```python
from build123d import *

# Parameters (mm, degrees)
SKETCH1_R                 = 1.5
SKETCH1_R_2               = 2.5
BATTERY_MOUNT_PLATE_DEPTH = 2.5
BATTERY_STRAP_SLOTS_DEPTH = 10
CUT_EXTRUDE1_DEPTH        = 10


with BuildPart() as part:
    # Sketch1 → battery mount plate (new body)
    with BuildSketch(Plane(origin=(0, 0, 0), x_dir=(1, 0, 0), z_dir=(0, 1, 0))):
        with BuildLine():
            Line((-145, 86), (145, 86))
            ThreePointArc((145, 86), (159.142135624, 80.142135624), (165, 66))
            Line((165, 66), (165, -66))
            ThreePointArc((165, -66), (159.142135624, -80.142135624), (145, -86))
            Line((145, -86), (-145, -86))
            ThreePointArc((-145, -86), (-159.142135624, -80.142135624), (-165, -66))
            Line((-165, -66), (-165, 66))
            ThreePointArc((-165, 66), (-159.142135624, 80.142135624), (-145, 86))
        make_face()
        with Locations(Location((143, 64, 0), (0, 0, 270))):
            Circle(SKETCH1_R, mode=Mode.SUBTRACT)
        with Locations(Location((-143, 64, 0), (0, 0, 90))):
            Circle(SKETCH1_R, mode=Mode.SUBTRACT)
        with Locations(Location((143, -64, 0), (0, 0, 90))):
            Circle(SKETCH1_R, mode=Mode.SUBTRACT)
        with Locations(Location((-143, -64, 0), (0, 0, 270))):
            Circle(SKETCH1_R, mode=Mode.SUBTRACT)
        with Locations(Location((-143, 20, 0), (0, 0, 270))):
            Circle(SKETCH1_R_2, mode=Mode.SUBTRACT)
        with Locations(Location((-143, -20, 0), (0, 0, 90))):
            Circle(SKETCH1_R_2, mode=Mode.SUBTRACT)
        with Locations(Location((143, 20, 0), (0, 0, 90))):
            Circle(SKETCH1_R_2, mode=Mode.SUBTRACT)
        with Locations(Location((143, -20, 0), (0, 0, 270))):
            Circle(SKETCH1_R_2, mode=Mode.SUBTRACT)
    extrude(amount=BATTERY_MOUNT_PLATE_DEPTH)

    # Sketch2 → battery strap slots (cut)
    with BuildSketch(Plane(origin=(0, 2.5, 0), x_dir=(1, 0, 0), z_dir=(0, 1, 0))):
        with BuildLine():
            Line((-25, 73), (-125, 73))
            ThreePointArc((-125, 73), (-127, 71), (-125, 69))
            Line((-125, 69), (-25, 69))
            ThreePointArc((-25, 69), (-23, 71), (-25, 73))
        make_face()
        with BuildLine():
            ThreePointArc((25, 73), (23, 71), (25, 69))
            Line((25, 69), (125, 69))
            ThreePointArc((125, 69), (127, 71), (125, 73))
            Line((125, 73), (25, 73))
        make_face()
        with BuildLine():
            ThreePointArc((25, 59), (23, 57), (25, 55))
            Line((25, 55), (125, 55))
            ThreePointArc((125, 55), (127, 57), (125, 59))
            Line((125, 59), (25, 59))
        make_face()
        with BuildLine():
            Line((-25, 59), (-125, 59))
            ThreePointArc((-125, 59), (-127, 57), (-125, 55))
            Line((-125, 55), (-25, 55))
            ThreePointArc((-25, 55), (-23, 57), (-25, 59))
        make_face()
        with BuildLine():
            Line((-25, -55), (-125, -55))
            ThreePointArc((-125, -55), (-127, -57), (-125, -59))
            Line((-125, -59), (-25, -59))
            ThreePointArc((-25, -59), (-23, -57), (-25, -55))
        make_face()
        with BuildLine():
            ThreePointArc((25, -55), (23, -57), (25, -59))
            Line((25, -59), (125, -59))
            ThreePointArc((125, -59), (127, -57), (125, -55))
            Line((125, -55), (25, -55))
        make_face()
        with BuildLine():
            ThreePointArc((25, -69), (23, -71), (25, -73))
            Line((25, -73), (125, -73))
            ThreePointArc((125, -73), (127, -71), (125, -69))
            Line((125, -69), (25, -69))
        make_face()
        with BuildLine():
            Line((-25, -69), (-125, -69))
            ThreePointArc((-125, -69), (-127, -71), (-125, -73))
            Line((-125, -73), (-25, -73))
            ThreePointArc((-25, -73), (-23, -71), (-25, -69))
        make_face()
    extrude(amount=-BATTERY_STRAP_SLOTS_DEPTH, mode=Mode.SUBTRACT)

    # Sketch3 → Cut-Extrude1 (cut)
    with BuildSketch(Plane(origin=(0, 2.5, 0), x_dir=(1, 0, 0), z_dir=(0, 1, 0))):
        with BuildLine():
            Line((-125, 40.910721278), (-125, 12))
            ThreePointArc((-125, 12), (-124.414213562, 10.585786438), (-123, 10))
            Line((-123, 10), (-85.829072643, 10))
            ThreePointArc((-85.829072643, 10), (-83.937326245, 11.35092715), (-84.601191416, 13.578704435))
            Line((-84.601191416, 13.578704435), (-121.772118773, 42.489425712))
            ThreePointArc((-121.772118773, 42.489425712), (-123.878702892, 42.707351798), (-125, 40.910721278))
        make_face()
        with BuildLine():
            Line((-84.601191416, -13.578704435), (-121.772118773, -42.489425712))
            ThreePointArc((-121.772118773, -42.489425712), (-123.878702892, -42.707351798), (-125, -40.910721278))
            Line((-125, -40.910721278), (-125, -12))
            ThreePointArc((-125, -12), (-124.414213562, -10.585786438), (-123, -10))
            Line((-123, -10), (-85.829072643, -10))
            ThreePointArc((-85.829072643, -10), (-83.937326245, -11.35092715), (-84.601191416, -13.578704435))
        make_face()
        with BuildLine():
            Line((-25, -40.910721278), (-25, -12))
            ThreePointArc((-25, -12), (-25.585786438, -10.585786438), (-27, -10))
            Line((-27, -10), (-64.170927357, -10))
            ThreePointArc((-64.170927357, -10), (-66.062673755, -11.35092715), (-65.398808584, -13.578704435))
            Line((-65.398808584, -13.578704435), (-28.227881227, -42.489425712))
            ThreePointArc((-28.227881227, -42.489425712), (-26.121297108, -42.707351798), (-25, -40.910721278))
        make_face()
        with BuildLine():
            Line((-65.398808584, 13.578704435), (-28.227881227, 42.489425712))
            ThreePointArc((-28.227881227, 42.489425712), (-26.121297108, 42.707351798), (-25, 40.910721278))
            Line((-25, 40.910721278), (-25, 12))
            ThreePointArc((-25, 12), (-25.585786438, 10.585786438), (-27, 10))
            Line((-27, 10), (-64.170927357, 10))
            ThreePointArc((-64.170927357, 10), (-66.062673755, 11.35092715), (-65.398808584, 13.578704435))
        make_face()
        with BuildLine():
            Line((-99.654825771, 42.489425712), (-50.345174229, 42.489425712))
            ThreePointArc((-50.345174229, 42.489425712), (-48.453427831, 41.138498563), (-49.117293002, 38.910721278))
            Line((-49.117293002, 38.910721278), (-73.772118773, 19.734745678))
            ThreePointArc((-73.772118773, 19.734745678), (-75, 19.313450112), (-76.227881227, 19.734745678))
            Line((-76.227881227, 19.734745678), (-100.882706998, 38.910721278))
            ThreePointArc((-100.882706998, 38.910721278), (-101.546572169, 41.138498563), (-99.654825771, 42.489425712))
        make_face()
        with BuildLine():
            Line((-49.117293002, -38.910721278), (-73.772118773, -19.734745678))
            ThreePointArc((-73.772118773, -19.734745678), (-75, -19.313450112), (-76.227881227, -19.734745678))
            Line((-76.227881227, -19.734745678), (-100.882706998, -38.910721278))
            ThreePointArc((-100.882706998, -38.910721278), (-101.546572169, -41.138498563), (-99.654825771, -42.489425712))
            Line((-99.654825771, -42.489425712), (-50.345174229, -42.489425712))
            ThreePointArc((-50.345174229, -42.489425712), (-48.453427831, -41.138498563), (-49.117293002, -38.910721278))
        make_face()
        with BuildLine():
            Line((76.227881227, -19.734745678), (100.882706998, -38.910721278))
            ThreePointArc((100.882706998, -38.910721278), (101.546572169, -41.138498563), (99.654825771, -42.489425712))
            Line((99.654825771, -42.489425712), (50.345174229, -42.489425712))
            ThreePointArc((50.345174229, -42.489425712), (48.453427831, -41.138498563), (49.117293002, -38.910721278))
            Line((49.117293002, -38.910721278), (73.772118773, -19.734745678))
            ThreePointArc((73.772118773, -19.734745678), (75, -19.313450112), (76.227881227, -19.734745678))
        make_face()
        with BuildLine():
            Line((76.227881227, 19.734745678), (100.882706998, 38.910721278))
            ThreePointArc((100.882706998, 38.910721278), (101.546572169, 41.138498563), (99.654825771, 42.489425712))
            Line((99.654825771, 42.489425712), (50.345174229, 42.489425712))
            ThreePointArc((50.345174229, 42.489425712), (48.453427831, 41.138498563), (49.117293002, 38.910721278))
            Line((49.117293002, 38.910721278), (73.772118773, 19.734745678))
            ThreePointArc((73.772118773, 19.734745678), (75, 19.313450112), (76.227881227, 19.734745678))
        make_face()
        with BuildLine():
            Line((25, 40.910721278), (25, 12))
            ThreePointArc((25, 12), (25.585786438, 10.585786438), (27, 10))
            Line((27, 10), (64.170927357, 10))
            ThreePointArc((64.170927357, 10), (66.062673755, 11.35092715), (65.398808584, 13.578704435))
            Line((65.398808584, 13.578704435), (28.227881227, 42.489425712))
            ThreePointArc((28.227881227, 42.489425712), (26.121297108, 42.707351798), (25, 40.910721278))
        make_face()
        with BuildLine():
            Line((65.398808584, -13.578704435), (28.227881227, -42.489425712))
            ThreePointArc((28.227881227, -42.489425712), (26.121297108, -42.707351798), (25, -40.910721278))
            Line((25, -40.910721278), (25, -12))
            ThreePointArc((25, -12), (25.585786438, -10.585786438), (27, -10))
            Line((27, -10), (64.170927357, -10))
            ThreePointArc((64.170927357, -10), (66.062673755, -11.35092715), (65.398808584, -13.578704435))
        make_face()
        with BuildLine():
            Line((125, -40.910721278), (125, -12))
            ThreePointArc((125, -12), (124.414213562, -10.585786438), (123, -10))
            Line((123, -10), (85.829072643, -10))
            ThreePointArc((85.829072643, -10), (83.937326245, -11.35092715), (84.601191416, -13.578704435))
            Line((84.601191416, -13.578704435), (121.772118773, -42.489425712))
            ThreePointArc((121.772118773, -42.489425712), (123.878702892, -42.707351798), (125, -40.910721278))
        make_face()
        with BuildLine():
            Line((84.601191416, 13.578704435), (121.772118773, 42.489425712))
            ThreePointArc((121.772118773, 42.489425712), (123.878702892, 42.707351798), (125, 40.910721278))
            Line((125, 40.910721278), (125, 12))
            ThreePointArc((125, 12), (124.414213562, 10.585786438), (123, 10))
            Line((123, 10), (85.829072643, 10))
            ThreePointArc((85.829072643, 10), (83.937326245, 11.35092715), (84.601191416, 13.578704435))
        make_face()
    extrude(amount=-CUT_EXTRUDE1_DEPTH, mode=Mode.SUBTRACT)


solid = part.part
```
Verification items for the finished model (mm, model axes). A direction names the side the tool comes from. Give positions to 0.01 mm unless a question says otherwise; leave off trailing zeros. One line per question, with ' | ' between items.
1) Thickness scan on line 1 along X through (y, z) = (1.05, 64); line 2 along Z through (x, y) = (-143, 2.05); line 3 along X through (y, z) = (0.6, -56.5). Record the ranges inside material, lowest first. Write a range as [from, to].
Result:
line 1: x = [-165, -144.5], [-141.5, 141.5], [144.5, 165] | line 2: z = [-86, -65.5], [-62.5, -22.5], [-17.5, 17.5], [22.5, 62.5], [65.5, 86] | line 3: x = [-165, -126.94], [-23.06, 23.06], [126.94, 165]
2) Set-up check for faces 1 (the cylindrical face through (158.986, 1.232, -80.297)), 2 (the flat face through (-102.926, 1.268, -27.832)): record each of +Z, -Z, +X, -X, +Y, -Y from which the full face is reachable in a straight line by a thin tool's end or side.
Result:
face 1: -Z, +X, +Y, -Y | face 2: +Y, -Y
3) Section check A-A on y = 1.8. State how many separate pieces and enclosed holes the cut face has, plus the area to 3 significant figures.
Result:
separate pieces: 1 | enclosed holes: 28 | area: 44,000 mm2
4) Gauge pin test, flat end, axial feed: pin 1 Ø3.5 at (x, z) = (143, 64) entering from -Y. Record the tip position at first contact, or that the pin passes through.
Result:
pin 1: stops at y = 0
